Geometry: final body of the model. Coordinates: model frame, mm. Give positions to 0.01 mm unless a question says otherwise; leave off trailing zeros. Loops run counter-clockwise (first coordinate to the right, second up) from the corner with the lowest first, then second, coordinate; pieces in that order, holes last. Notation, with made-up numbers: (17, 68) - (28, 68) arc R24 ccw to (28, 96) - close; hole circle Ø4 at (62.5, 2). An arc over 180 degrees is marked (long way). Use one line per item in the form item = value.
```python
from build123d import *

# Parameters (mm, degrees)
F0_W     = 105
F0_H     = 30
F1_DEPTH = 2.14
F2_R     = 2.6
F3_R     = 1.5
F4_DEPTH = 2.14
F5_R     = 0.3


with BuildPart() as f1:
    # F0 (on Top) → F1 (new body)
    with BuildSketch(Plane.XY):
        Rectangle(F0_W, F0_H)
    extrude(amount=F1_DEPTH)

    # F2
    f2_edges = [f1.edges().sort_by_distance(p)[0] for p in [
        (-52.5, -15, 1.07),
        (-52.5, 15, 1.07),
        (52.5, 15, 1.07),
        (52.5, -15, 1.07),
    ]]
    fillet(f2_edges, radius=F2_R)

    # F3 (on face) → F4 (cut, through all)
    with BuildSketch(Plane.XY.offset(2.14)):
        with Locations((-49, 11.3)):
            Circle(F3_R)
        with Locations((-49, -11.3)):
            Circle(F3_R)
        with Locations((49, -11.3)):
            Circle(F3_R)
        with Locations((49, 11.3)):
            Circle(F3_R)
    extrude(amount=-F4_DEPTH, mode=Mode.SUBTRACT)

    # F5
    f5_edges = [f1.edges().sort_by_distance(p)[0] for p in [
        (52.5, 0, 2.14),
        (51.738478, -14.238478, 2.14),
        (51.738478, 14.238478, 2.14),
        (0, -15, 2.14),
        (0, 15, 2.14),
        (-51.738478, -14.238478, 2.14),
        (-51.738478, 14.238478, 2.14),
        (-52.5, 0, 2.14),
        (-50.5, -11.3, 2.14),
        (47.5, -11.3, 2.14),
        (-50.5, 11.3, 2.14),
        (47.5, 11.3, 2.14),
    ]]
    fillet(f5_edges, radius=F5_R)


solid = f1.part
```
(1) Material intervals for L1, parallel to Y at x = -49, z = 0.8; L2, parallel to X at y = 5, z = 1.95, sorted ascending. Write a range as from..to.
Solution:
L1 = -15..-12.8, -9.8..9.8, 12.8..15
L2 = -52.48..52.48
(2) Cut plane A-A (y = 11.3). Return the cut outline in (x, z), plus the area to 3 significant figures.
Solution:
outline = (-52.5, 0) - (-50.5, 0) - (-50.5, 1.84) arc R0.3 ccw to (-50.8, 2.14) - (-52.2, 2.14) arc R0.3 ccw to (-52.5, 1.84) - close; (-47.5, 0) - (47.5, 0) - (47.5, 1.84) arc R0.3 ccw to (47.2, 2.14) - (-47.2, 2.14) arc R0.3 ccw to (-47.5, 1.84) - close; (50.5, 0) - (52.5, 0) - (52.5, 1.84) arc R0.3 ccw to (52.2, 2.14) - (50.8, 2.14) arc R0.3 ccw to (50.5, 1.84) - close
area = 212 mm2
(3) Cut plane B-B (x = -49). Return the cut outline in (y, z), plus the area to 3 significant figures.
Solution:
outline = (-15, 0) - (-12.8, 0) - (-12.8, 1.84) arc R0.3 ccw to (-13.1, 2.14) - (-14.7, 2.14) arc R0.3 ccw to (-15, 1.84) - close; (-9.8, 0) - (9.8, 0) - (9.8, 1.84) arc R0.3 ccw to (9.5, 2.14) - (-9.5, 2.14) arc R0.3 ccw to (-9.8, 1.84) - close; (12.8, 0) - (15, 0) - (15, 1.84) arc R0.3 ccw to (14.7, 2.14) - (13.1, 2.14) arc R0.3 ccw to (12.8, 1.84) - close
area = 51.2 mm2
(4) Pin query (flat end, axial travel): P1, Ø3.5, axis at x = 49, y = 11.3, coming from the +Z side. Return the tip coordinate at first contact, or that it passes through.
Solution:
P1 = 2.14
(5) Pull-direction query (Y, two-part tool) for faces 1 (the face through (47.8, -12.2, 0.9)), 2 (the face through (51.759, 14.218, 0.933)), 3 (the face through (-1, 0, 2.14)); classes: released by +Y, released by -Y, zero draft, split by the parting line, or undercut.
Solution:
face_1 = undercut
face_2 = released by +Y
face_3 = zero draft
